Job drawing, mm, ordinate dimensions from the low corner. One solid piece. Give positions to 0.01 mm unless a question says otherwise; leave off trailing zeros. Order: outer loops, then holes, each group sorted by start corner. A loop starts at its lowest first (then second) coordinate and runs counter-clockwise, first axis right, second up. Notation, with made-up numbers: (12, 32.25) -> (71, 32.25) arc R26 ccw to (71, 65.25) -> close; hole circle Ø1 at (56.5, -22.5). An arc over 180 degrees is marked (long way). Use CSV: the item, a comma, the result in double quotes. Start each with the question number.
1. Pull direction X, two halves, no side cores. Call the marked faces 1 and 2: released by +X, released by -X, zero draft, split by the parting line, or undercut.
2. Cut at A-A on x = 20.5. List the corners of the cut face in (y, z).
3. Drop a flat-ended pin along its axis: pin 1 (1.5 mm diameter, centred on x = 26, z = 2.5, fed in from +Y). Give the stop position or say it passes through.
4. Cut at C-C on z = 2.3. List the corners of the cut face in (x, y), then the cut area to 3 significant figures.
5. Cut at D-D on x = 35. List the corners of the cut face in (y, z).
6. Wall check: line 1 (Y direction, x = 35, z = 0.7); line 2 (X direction, y = 27, z = 0.5); line 3 (Y direction, x = 20.5, z = 1.4). Give the ranges that are in metal, low to high. Write a range as from..to.
7. Cut at B-B on y = 28.5. List the corners of the cut face in (x, z), then the cut area to 3 significant figures.
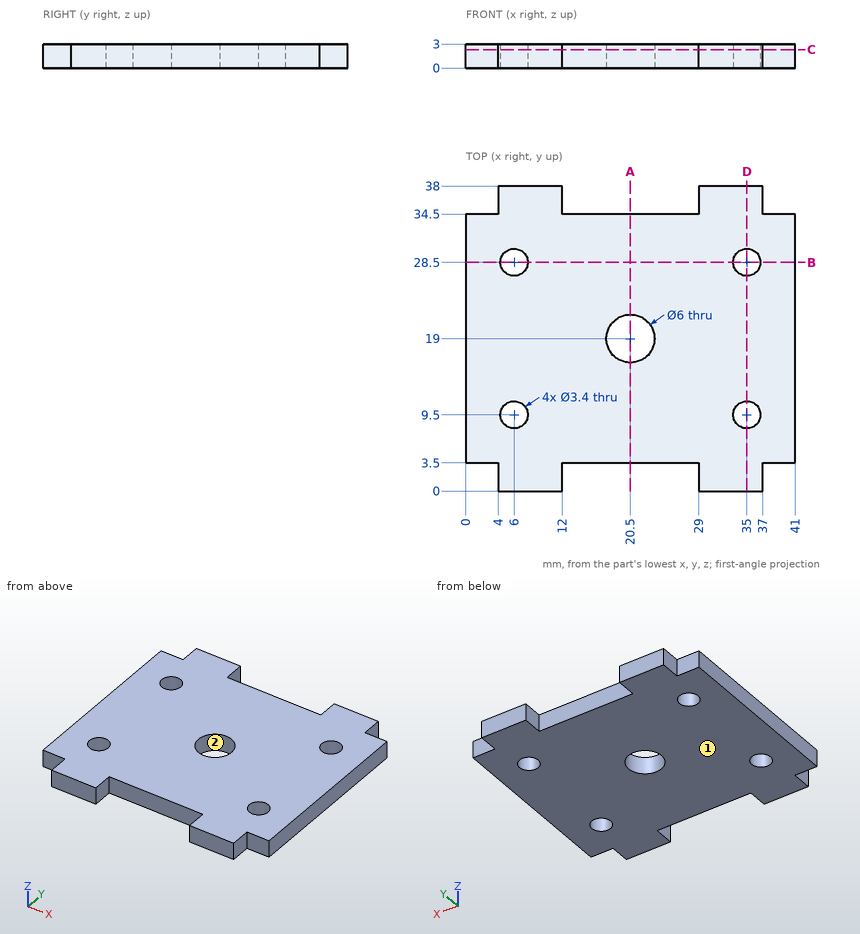
Verdict:
1,face 1,"zero draft"
1,face 2,"undercut"
2,outline,"(3.5, 0) -> (16, 0) -> (16, 3) -> (3.5, 3) -> close; (22, 0) -> (34.5, 0) -> (34.5, 3) -> (22, 3) -> close"
3,pin 1,"y = 34.5"
4,outline,"(0, 3.5) -> (4, 3.5) -> (4, 0) -> (12, 0) -> (12, 3.5) -> (29, 3.5) -> (29, 0) -> (37, 0) -> (37, 3.5) -> (41, 3.5) -> (41, 34.5) -> (37, 34.5) -> (37, 38) -> (29, 38) -> (29, 34.5) -> (12, 34.5) -> (12, 38) -> (4, 38) -> (4, 34.5) -> (0, 34.5) -> close; hole circle Ø3.4 at (6, 9.5); hole circle Ø3.4 at (6, 28.5); hole circle Ø6 at (20.5, 19); hole circle Ø3.4 at (35, 9.5); hole circle Ø3.4 at (35, 28.5)"
4,area,"1,320 mm^2"
5,outline,"(0, 0) -> (7.8, 0) -> (7.8, 3) -> (0, 3) -> close; (11.2, 0) -> (26.8, 0) -> (26.8, 3) -> (11.2, 3) -> close; (30.2, 0) -> (38, 0) -> (38, 3) -> (30.2, 3) -> close"
6,line 1,"0..7.8, 11.2..26.8, 30.2..38"
6,line 2,"0..5.2, 6.8..34.2, 35.8..41"
6,line 3,"3.5..16, 22..34.5"
7,outline,"(0, 0) -> (4.3, 0) -> (4.3, 3) -> (0, 3) -> close; (7.7, 0) -> (33.3, 0) -> (33.3, 3) -> (7.7, 3) -> close; (36.7, 0) -> (41, 0) -> (41, 3) -> (36.7, 3) -> close"
7,area,"103 mm^2"
